from build123d import *

# Parameters (mm, degrees)
SALIENTE_EXTRUIR1_DEPTH      = 3
CORTAR_EXTRUIR1_DEPTH        = 130.745905523
CORTAR_EXTRUIR1_DEPTH_BACK   = 130.745905523
CROQUIS2_R                   = 4.5
TALADRO_DE_MARGEN_PARA_M42_D = 4.5
TALADRO_DE_MARGEN_PARA_M41_D = 4.5


with BuildPart() as part:
    # Croquis1 → Saliente-Extruir1 (new, symmetric)
    with BuildSketch(Plane(origin=(0, 0, 0), x_dir=(1, 0, 0), z_dir=(0, 1, 0))):
        Polygon((-54, -109), (-25, -109), (-25, -115), (25, -115), (25, -109), (54, -109), (54, -30), (60, -30), (60, 30), (54, 30), (54, 109), (25, 109), (25, 115), (-25, 115), (-25, 109), (-54, 109), (-54, 30), (-60, 30), (-60, -30), (-54, -30), align=None)
    extrude(amount=SALIENTE_EXTRUIR1_DEPTH, both=True)

    # Croquis2 → Cortar-Extruir1 (cut, two sides: drawn at the far end of the back side and taken through both)
    with BuildSketch(Plane(origin=(0, 0, 0), x_dir=(1, 0, 0), z_dir=(0, 1, 0)).offset(-CORTAR_EXTRUIR1_DEPTH_BACK)):
        with Locations(Location((0, -65, 0), (0, 0, 270))):
            Circle(CROQUIS2_R)
    extrude(amount=CORTAR_EXTRUIR1_DEPTH + CORTAR_EXTRUIR1_DEPTH_BACK, mode=Mode.SUBTRACT)

    # Taladro de margen para M42 (through all)
    with Locations(Plane(origin=(0, 3, 0), x_dir=(1, 0, 0), z_dir=(0, 1, 0))):
        with Locations((12.5, -77.5), (-12.5, -77.5), (12.5, -52.5), (-12.5, -52.5)):
            Hole(TALADRO_DE_MARGEN_PARA_M42_D / 2)

    # Taladro de margen para M41 (through all)
    with Locations(Plane(origin=(0, -3, 0), x_dir=(-1, 0, 0), z_dir=(0, -1, 0))):
        with Locations((40, 80), (-40, 80), (40, -65), (-40, -65)):
            Hole(TALADRO_DE_MARGEN_PARA_M41_D / 2)


solid = part.part
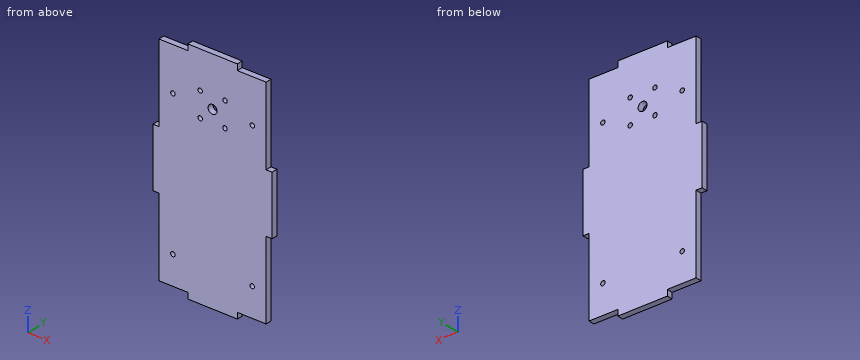
Check sheet for the modelled part. Datum: model origin and axes. Units: mm. Give positions to 0.01 mm unless a question says otherwise; leave off trailing zeros. Write each loop counter-clockwise with the first axis right and the second up, starting at its lowest first coordinate (ties: lowest second). Pieces come first, ordered by that corner, then holes. Notation, with made-up numbers: M 19.25,45.25 L 68.25,45.25 A27 cw 68.25,74.25 Z; hole C -22,29.25 d10. An arc over 180 degrees is marked long. Use one line per item in the form item = value.
(1) Section check A-A on z = 65. Record the boundary of the cut face in (x, y).
Answer block:
outline = M -54,-3 L -42.25,-3 L -42.25,3 L -54,3 Z; M -37.75,-3 L -4.5,-3 L -4.5,3 L -37.75,3 Z; M 4.5,-3 L 37.75,-3 L 37.75,3 L 4.5,3 Z; M 42.25,-3 L 54,-3 L 54,3 L 42.25,3 Z
(2) Section check D-D on x = 0. Record the boundary of the cut face in (y, z).
Answer block:
outline = M -3,-115 L 3,-115 L 3,60.5 L -3,60.5 Z; M -3,69.5 L 3,69.5 L 3,115 L -3,115 Z
(3) Depth check by flat-ended pin: P1, Ø5, axis at x = 12.5, z = 52.5, coming from the +Y side; P2, Ø3, axis at y = 0, z = -55.5, coming from the -X side; P3, Ø1.8, axis at x = 56, y = 0.5, coming from the +Z side; P4, Ø1, axis at x = -34, y = -2.5, coming from the -Z side. Enter the tip coordinate at first touch or a pass-through.
Answer block:
P1 = 3
P2 = -54
P3 = 30
P4 = -109
(4) Section check B-B on x = -12.5. Record the boundary of the cut face in (y, z), plus the area to 3 significant figures.
Answer block:
outline = M -3,-115 L 3,-115 L 3,50.25 L -3,50.25 Z; M -3,54.75 L 3,54.75 L 3,75.25 L -3,75.25 Z; M -3,79.75 L 3,79.75 L 3,115 L -3,115 Z
area = 1,330 mm2
(5) Material ranges on line 1 along X through (y, z) = (-1.1, 52.5); line 2 along Z through (x, y) = (-40, 1.15); line 3 along Z through (x, y) = (12.5, 0.2), recorded low to high.
Answer block:
line_1 = -54 to -14.75, -10.25 to 10.25, 14.75 to 54
line_2 = -109 to -82.25, -77.75 to 62.75, 67.25 to 109
line_3 = -115 to 50.25, 54.75 to 75.25, 79.75 to 115
(6) Section check C-C on y = 1.3. State how many separate pieces and enclosed holes the cut face has, plus the area to 3 significant figures.
Answer block:
separate_pieces = 1
enclosed_holes = 9
area = 24,700 mm2
